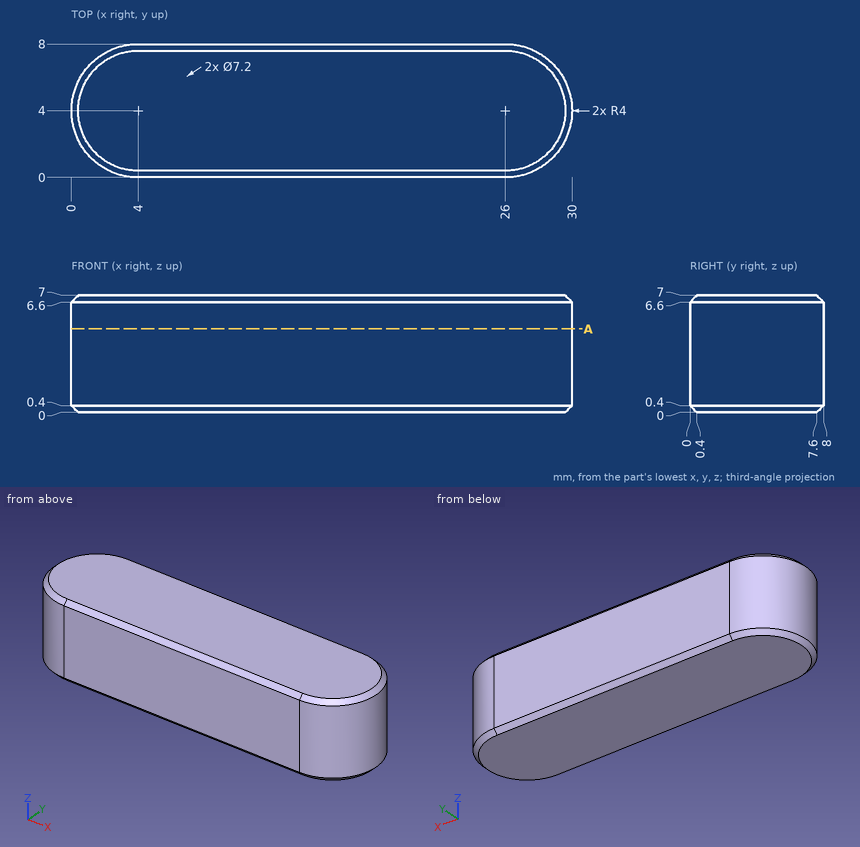
Study the drawing (mm; zero at the part's minimum x, y, z) and answer. Round coordinates to 2 decimals unless told otherwise and drop trailing zeros. Order: outer loops, then holes, each group sorted by start corner. A loop starts at its lowest first (then second) coordinate and runs counter-clockwise, first axis right, second up. Notation, with made-up numbers: M -19.75,79.25 L -8.75,79.25 A12 ccw -8.75,99.25 Z; hole C -23,75 d6. An arc over 180 degrees is marked long. One line per item, written item: value.
Q1. Find section A-A on z = 5. Write down the section's boundary in (x, y).
Derived:
outline: M 4,0 L 26,0 A4 ccw 26,8 L 4,8 A4 ccw Z
Q2. Flat-ended cylindrical pins translate along their axes: pin 1 (2 mm diameter, centred on y = 5.5, z = 5, fed in from +X); pin 2 (1 mm diameter, centred on y = 2.5, z = 6, fed in from -X). Find the tip coordinate at first contact, or state that the pin passes through.
Derived:
pin 1: x = 29.97
pin 2: x = 0.13
Q3. Straight lines are drawn through the part: line 1 (X direction, y = 4.25, z = 6.25); line 2 (X direction, y = 6.5, z = 2.75); line 3 (Y direction, x = 26.75, z = 3.75). For each, find the intervals that lie inside material, in ascending order.
Derived:
line 1: 0.01 to 29.99
line 2: 0.88 to 29.12
line 3: 0.07 to 7.93
